The model under review builds one solid part; all positions refer to its coordinate system, in mm. Round coordinates to 2 decimals unless told otherwise and drop trailing zeros. Loops run counter-clockwise (first coordinate to the right, second up) from the corner with the lowest first, then second, coordinate; pieces in that order, holes last. Notation, with made-up numbers: M 60,59 L 66,59 A25 cw 66,85 Z; hole C 72.25,3 d3. An arc over 180 degrees is marked long. Return JSON: item names as keys, results as strings. Group by question number.
Q1. Consider section A-A (y = 6). State the section outline as (x, z) points, and give its area (3 significant figures).
Q2. Consider section B-B (z = 3.75). State the section outline as (x, y) points (1 decimal), and give its area (3 significant figures).
Q3. To check wall thickness, follow line 1 along Y through (x, z) = (37, 7.5); line 2 along X through (y, z) = (7, 4.75); line 3 along Y through (x, z) = (38, 2). State the ranges of each line that lie inside material, in increasing order.
Q4. Consider section C-C (x = 13). State the section outline as (y, z) points.
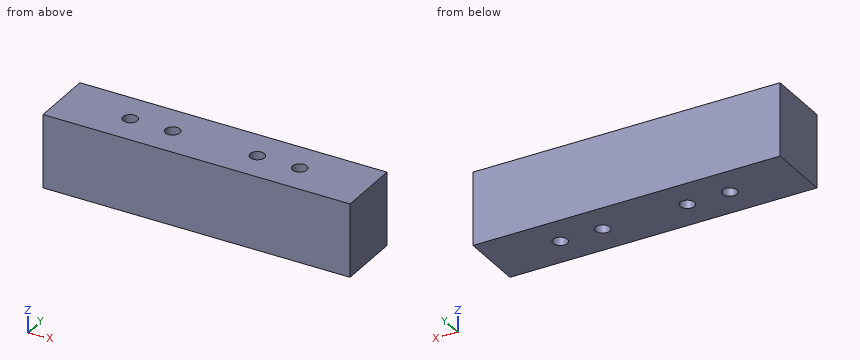
Autodesk Inventor part; units mm, degrees
ref_plane "YZ Plane" through (0, 0, 0) normal (1, 0, 0) x (0, 1, 0)
ref_plane "XZ Plane" through (0, 0, 0) normal (0, 1, 0) x (-1, 0, 0)
ref_plane "XY Plane" through (0, 0, 0) normal (0, 0, 1) x (1, 0, 0)
sketch "Sketch1" plane through (0, 0, 0) normal (0, 0, 1) x (1, 0, 0)
  circle A0 centre (13, 6) radius 1.3525
  circle A1 centre (21, 6) radius 1.3525
  circle A2 centre (37, 6) radius 1.3525
  circle A3 centre (45, 6) radius 1.3525
  line L0 (0, 0) -> (58, 0)
  line L1 (58, 0) -> (58, 12)
  line L2 (0, 12) -> (58, 12)
  line L3 (0, 12) -> (0, 0)
  point P0 (29, 6)
extrude "Extrusion1" add sketch "Sketch1" along normal blind 13.843
properties part number "Motor Spacer"
Values:
{
 "1": {"outline": "M 0,0 L 11.65,0 L 11.65,13.84 L 0,13.84 Z; M 14.35,0 L 19.65,0 L 19.65,13.84 L 14.35,13.84 Z; M 22.35,0 L 35.65,0 L 35.65,13.84 L 22.35,13.84 Z; M 38.35,0 L 43.65,0 L 43.65,13.84 L 38.35,13.84 Z; M 46.35,0 L 58,0 L 58,13.84 L 46.35,13.84 Z", "area": "653 mm2"},
 "2": {"outline": "M 0,0 L 58,0 L 58,12 L 0,12 Z; hole C 13,6 d2.7; hole C 21,6 d2.7; hole C 37,6 d2.7; hole C 45,6 d2.7", "area": "673 mm2"},
 "3": {"line 1": "y = 0 to 4.65, 7.35 to 12", "line 2": "x = 0 to 12.09, 13.91 to 20.09, 21.91 to 36.09, 37.91 to 44.09, 45.91 to 58", "line 3": "y = 0 to 5.09, 6.91 to 12"},
 "4": {"outline": "M 0,0 L 4.65,0 L 4.65,13.84 L 0,13.84 Z; M 7.35,0 L 12,0 L 12,13.84 L 7.35,13.84 Z"}
}
